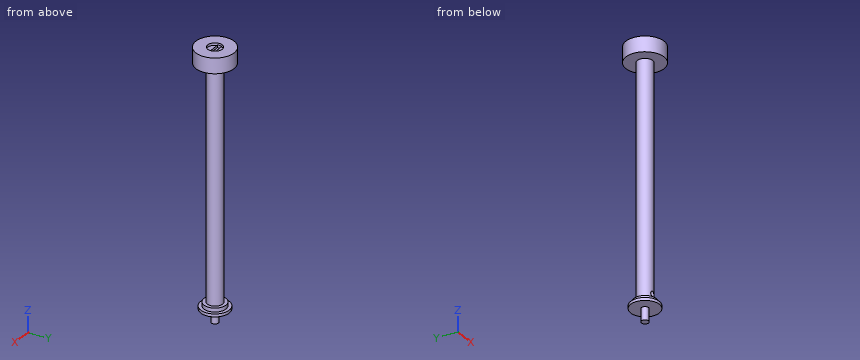
from build123d import *

# Parameters (mm, degrees)
SKETCH1_R                    = 1.5
SOCKET_PIN_DEPTH             = 5.5
SKETCH2_R                    = 6
MAST_FLANGE_DEPTH            = 1.2
SKETCH3_R                    = 4.6
MAST_FLANGE_STEP_DEPTH       = 1.6
SKETCH4_R                    = 3.2
MAST_TUBE_DEPTH              = 97.8
SKETCH5_R                    = 8
BEACON_BASE_DEPTH            = 6.4
SKETCH6_R                    = 5.5
SOLDER_CHAMBER_DEPTH         = 1.8
SKETCH7_W                    = 6.4
SKETCH7_H                    = 1.8
LED_LEG_SLOT_DEPTH           = 0.7
SKETCH8_R                    = 3.05
LED_FLANGE_COUNTERBORE_DEPTH = 0.7
SKETCH9_R                    = 1.1
WIRE_CHANNEL_DEPTH           = 49
SKETCH10_R                   = 1.1
WIRE_EXIT_DEPTH              = 2.25


with BuildPart() as part:
    # Sketch1 → Socket_pin (new body)
    with BuildSketch(Plane.XY.offset(54.6)):
        with Locations((172, 45)):
            Circle(SKETCH1_R)
    extrude(amount=SOCKET_PIN_DEPTH)

    # Sketch2 → Mast_flange (add)
    with BuildSketch(Plane.XY.offset(60)):
        with Locations((172, 45)):
            Circle(SKETCH2_R)
    extrude(amount=MAST_FLANGE_DEPTH)

    # Sketch3 → Mast_flange_step (add)
    with BuildSketch(Plane.XY.offset(61.2)):
        with Locations((172, 45)):
            Circle(SKETCH3_R)
    extrude(amount=MAST_FLANGE_STEP_DEPTH)

    # Sketch4 → Mast_tube (add)
    with BuildSketch(Plane.XY.offset(62.7)):
        with Locations((172, 45)):
            Circle(SKETCH4_R)
    extrude(amount=MAST_TUBE_DEPTH)

    # Sketch5 → Beacon_base (add)
    with BuildSketch(Plane.XY.offset(160)):
        with Locations((172, 45)):
            Circle(SKETCH5_R)
    extrude(amount=BEACON_BASE_DEPTH)

    # Sketch6 → Solder_chamber (cut, symmetric)
    with BuildSketch(Plane.XY.offset(162.6)):
        with Locations((172, 45)):
            Circle(SKETCH6_R)
    extrude(amount=SOLDER_CHAMBER_DEPTH, both=True, mode=Mode.SUBTRACT)

    # Sketch7 → LED_leg_slot (cut, symmetric)
    with BuildSketch(Plane.XY.offset(164.9)):
        with Locations((172, 45)):
            Rectangle(SKETCH7_W, SKETCH7_H)
    extrude(amount=LED_LEG_SLOT_DEPTH, both=True, mode=Mode.SUBTRACT)

    # Sketch8 → LED_flange_counterbore (cut, symmetric)
    with BuildSketch(Plane.XY.offset(166.1)):
        with Locations((172, 45)):
            Circle(SKETCH8_R)
    extrude(amount=LED_FLANGE_COUNTERBORE_DEPTH, both=True, mode=Mode.SUBTRACT)

    # Sketch9 → Wire_channel (cut, symmetric)
    with BuildSketch(Plane.XY.offset(112)):
        with Locations((172, 45)):
            Circle(SKETCH9_R)
    extrude(amount=WIRE_CHANNEL_DEPTH, both=True, mode=Mode.SUBTRACT)

    # Sketch10 → Wire_exit (cut, symmetric)
    with BuildSketch(Plane(origin=(0, 42.75, 0), x_dir=(1, 0, 0), z_dir=(0, 1, 0))):
        with Locations(Location((172, -65, 0), (0, 0, 270))):
            Circle(SKETCH10_R)
    extrude(amount=WIRE_EXIT_DEPTH, both=True, mode=Mode.SUBTRACT)


solid = part.part
Source: CAD feature listing. Evaluate the final solid. Frame: model axes, mm. Round coordinates to 2 decimals unless told otherwise and drop trailing zeros. Write each loop counter-clockwise with the first axis right and the second up, starting at its lowest first coordinate (ties: lowest second). Pieces come first, ordered by that corner, then holes. Notation, with made-up numbers: M -14,-8 L 41,-8 A15 cw 41,19 Z; hole C 78.5,1.25 d4. An arc over 180 degrees is marked long. One line per item, written item: value. Start each with the question number.
Item 1: Section query B-B (y = 52). Return the cut outline in (x, z), plus the area to 3 significant figures.
Item 2: Ray query, L1, parallel to Z at x = 168.5, y = 44; L2, parallel to Z at x = 172, y = 42.5; L3, parallel to Y at x = 172, z = 163.4. Return the intervals inside material, ascending. Write a range as from..to.
Item 3: Section query C-C (z = 65). Return the cut outline in (x, y) (3 decimals).
Item 4: Pin query (flat end, axial travel): pin 1 (4 mm diameter, centred on y = 46.5, z = 79, fed in from +X); pin 2 (3 mm diameter, centred on x = 168.5, y = 45, fed in from -Z); pin 3 (8 mm diameter, centred on y = 44, z = 106.5, fed in from -X). Return the tip coordinate at first contact, or that it passes through.
Item 5: Section query A-A (z = 81.5). Return the cut outline in (x, y).
Result set:
1. outline: M 168.13,160 L 175.87,160 L 175.87,166.4 L 168.13,166.4 Z
1. area: 49.6 mm²
2. L1: z = 60..62.8, 160..160.8, 164.4..166.4
2. L2: z = 60..63.9, 66.1..160.8, 164.4..165.4
2. L3: y = 37..39.5, 50.5..53
3. outline: M 170.9,41.995 L 170.9,45 A1.1 cw 173.1,45 L 173.1,41.995 A3.2 ccw long Z
4. pin 1: stops at x = 175.2
4. pin 2: stops at z = 60
4. pin 3: stops at x = 168.8
5. outline: C 172,45 d6.4; hole C 172,45 d2.2
